Part print with two shaded views. Sizes in mm from the minimum x, y, z corner. Coordinates: 2 decimals unless noted, no trailing zeros. Loops run counter-clockwise (first coordinate to the right, second up) from the corner with the lowest first, then second, coordinate; pieces in that order, holes last.
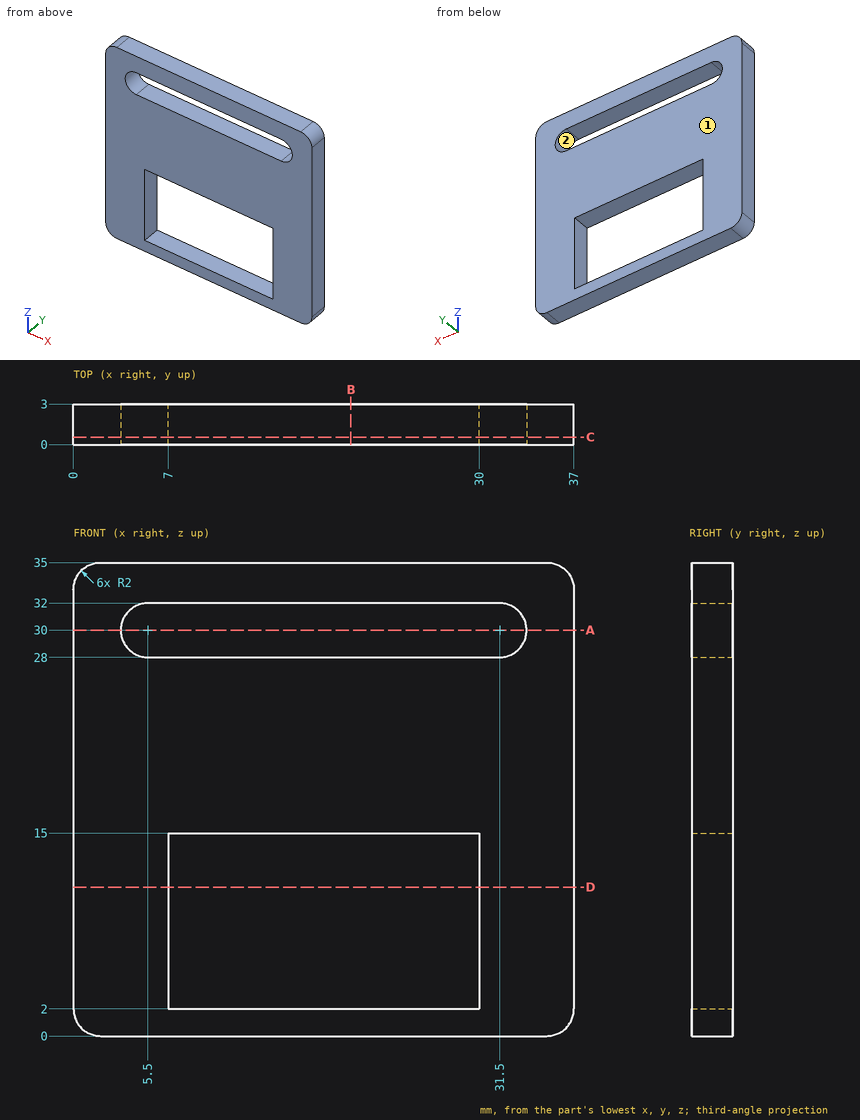
Q1. Slice it at B-B (x = 20.5). List the corners of the cut face in (y, z), and give its area (3 significant figures).
Answers:
outline: (0, 0) - (3, 0) - (3, 2) - (0, 2) - close; (0, 15) - (3, 15) - (3, 28) - (0, 28) - close; (0, 32) - (3, 32) - (3, 35) - (0, 35) - close
area: 54.0 mm2
Q2. Slice it at D-D (z = 11). List the corners of the cut face in (x, y), and give its area (3 significant figures).
Answers:
outline: (0, 0) - (7, 0) - (7, 3) - (0, 3) - close; (30, 0) - (37, 0) - (37, 3) - (30, 3) - close
area: 42.0 mm2
Q3. Mould opens along X. For the marked faces 1 and 2 say: +X half, -X half, draft (parallel to the pull), parting line (faces both ways), or undercut.
Answers:
face 1: draft
face 2: undercut
Q4. Drill centre lines: line 1 (Z direction, x = 24, y = 2.4); line 2 (X direction, y = 0.6, z = 3.5); line 3 (Z direction, x = 5, y = 1.35). Where is each one in solid material? Low to high.
Answers:
line 1: z = 0 to 2, 15 to 28, 32 to 35
line 2: x = 0 to 7, 30 to 37
line 3: z = 0 to 28.06, 31.94 to 35
Q5. Slice it at A-A (z = 30). List the corners of the cut face in (x, y).
Answers:
outline: (0, 0) - (3.5, 0) - (3.5, 3) - (0, 3) - close; (33.5, 0) - (37, 0) - (37, 3) - (33.5, 3) - close
Q6. Slice it at C-C (y = 0.55). List the corners of the cut face in (x, z), and give its area (3 significant figures).
Answers:
outline: (0, 2) arc R2 ccw to (2, 0) - (35, 0) arc R2 ccw to (37, 2) - (37, 33) arc R2 ccw to (35, 35) - (2, 35) arc R2 ccw to (0, 33) - close; hole (5.5, 28) - (31.5, 28) arc R2 ccw to (31.5, 32) - (5.5, 32) arc R2 ccw to start; hole (7, 2) - (30, 2) - (30, 15) - (7, 15) - close
area: 876 mm2
